Autodesk Fusion 360 part; units mm, degrees
sketch "Sketch1" plane through (0, 0, 0) normal (0, 1, 0) x (1, 0, 0)
  circle A0 centre (0, 0) radius 4
  dimension "d1" = 8
extrude "Extrude1" add sketch "Sketch1" along normal blind 11
sketch "Sketch2" plane through (0, 0, 0) normal (1, 0, 0) x (0, 1, 0)
  line L0 (0, -4) -> (0, 4)
  line L1 (0, 0) -> (0, 0.8)
  line L2 (0, 0.8) -> (0, -0.8)
  line L3 (0, 0) -> (0, 0.8)
  line L4 (0, 0.8) -> (0, -0.8)
  line L5 (0, 0.8) -> (1.8, 0.8)
  line L6 (1.8, 0.8) -> (1.8, -0.8)
  line L7 (1.8, -0.8) -> (0, -0.8)
  dimension "d6" = 0.8
  dimension "d7" = 1.6
  dimension "d8" = 1.8
  dimension "d9" = 1.6
extrude "Extrude2" cut sketch "Sketch2" along normal blind 5.3 and the other way blind 4.5
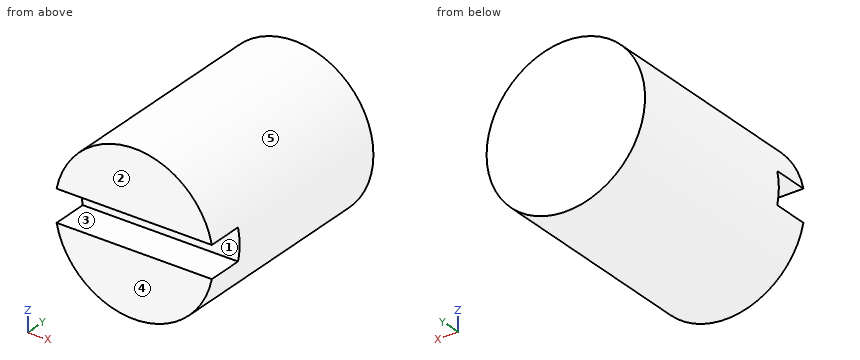
Read the model definition and answer for the solid it produces. Units are mm, in the model's axes. Face numbers are marked on the shaded views. A direction names the side the tool comes from. Coordinates: 2 decimals unless noted, no trailing zeros. Write each loop counter-clockwise with the first axis right and the second up, starting at its lowest first coordinate (ties: lowest second). Pieces come first, ordered by that corner, then holes. Notation, with made-up numbers: M 70,53.25 L 119,53.25 A29 cw 119,84.25 Z; hole C 5.5,-8 d5. An arc over 180 degrees is marked long. Use a Markdown table: item, result.
Q1. The part is cut by section A-A, the plane x = 0. Write down the section's boundary in (y, z).
Answer block:
| item | result |
|---|---|
| outline | M 0,-4 L 11,-4 L 11,4 L 0,4 L 0,0.8 L 1.8,0.8 L 1.8,-0.8 L 0,-0.8 Z |
Q2. Which of the six approach directions +Z, -Z, +X, -X, +Y, -Y give full straight-line access (tool end or side, diameter ignored) to the marked faces 1 and 2?
Answer block:
| item | result |
|---|---|
| face 1 | +X, -X, -Y |
| face 2 | +Z, -Z, +X, -X, -Y |
Q3. The part is cut by section C-C, the plane z = 0. Write down the section's boundary in (x, y), then the cut area to 3 significant figures.
Answer block:
| item | result |
|---|---|
| outline | M -4,1.8 L 4,1.8 L 4,11 L -4,11 Z |
| area | 73.6 mm2 |
Q4. Each of these flat-tipped pins is pushed along its axis until it touches: pin 1 Ø3 at (y, z) = (4.5, -3) entering from +X; pin 2 Ø1 at (y, z) = (9, -2.5) entering from +X; pin 3 Ø0.5 at (x, y) = (-1, 1) entering from -Z. Where does it stop, or does it pass through?
Answer block:
| item | result |
|---|---|
| pin 1 | stops at x = 3.71 |
| pin 2 | stops at x = 3.46 |
| pin 3 | stops at z = -3.93 |
Q5. The part is cut by section B-B, the plane y = 2.5. Write down the section's boundary in (x, z).
Answer block:
| item | result |
|---|---|
| outline | C 0,0 d8 |
Q6. The part is cut by section D-D, the plane x = 1. Write down the section's boundary in (y, z), then the cut area to 3 significant figures.
Answer block:
| item | result |
|---|---|
| outline | M 0,-3.87 L 11,-3.87 L 11,3.87 L 0,3.87 L 0,0.8 L 1.8,0.8 L 1.8,-0.8 L 0,-0.8 Z |
| area | 82.3 mm2 |
Q7. Straight lines are drawn through the part: L1, parallel to Y at x = 3, z = 0.5; L2, parallel to Z at x = -1, y = 3.5; L3, parallel to X at y = 7.25, z = -2.5. For each, find the intervals that lie inside material, in ascending order. Write a range as [from, to].
Answer block:
| item | result |
|---|---|
| L1 | y = [1.8, 11] |
| L2 | z = [-3.87, 3.87] |
| L3 | x = [-3.12, 3.12] |
Q8. Determine the mould class of the marked faces 3, 4 and 5 for opening direction Z: released by +Z, released by -Z, zero draft, split by the parting line, or undercut.
Answer block:
| item | result |
|---|---|
| face 3 | undercut |
| face 4 | zero draft |
| face 5 | split by the parting line |
